Autodesk Inventor part; units mm, degrees
ref_plane "YZ Plane" through (0, 0, 0) normal (1, 0, 0) x (0, 1, 0)
ref_plane "XZ Plane" through (0, 0, 0) normal (0, 1, 0) x (-1, 0, 0)
ref_plane "XY Plane" through (0, 0, 0) normal (0, 0, 1) x (1, 0, 0)
sketch "Sketch1" plane through (0, 0, 0) normal (0, 0, 1) x (1, 0, 0)
  line L0 (-10.16, 7.62) -> (-15.748, 7.62)
  line L1 (-15.748, 7.62) -> (-15.748, 18.034)
  line L2 (-15.748, 18.034) -> (-23.368, 18.034)
  line L3 (-23.368, 18.034) -> (-23.368, 7.62)
  line L4 (-23.368, 7.62) -> (-105.283, 7.62)
  line L5 (-105.283, 7.62) -> (-105.283, 18.034)
  line L6 (-105.283, 18.034) -> (-112.903, 18.034)
  line L7 (-112.903, 18.034) -> (-112.903, 7.62)
  line L8 (-112.903, 7.62) -> (-123.571, 7.62)
  line L9 (-123.571, 7.62) -> (-123.571, 31.75)
  line L10 (-123.571, 31.75) -> (-133.731, 31.75)
  circle A0 centre (-109.093, 14.224) radius 1.778
  line L11 (-133.731, 31.75) -> (-133.731, 0)
  line L12 (-133.731, 0) -> (0, 0)
  circle A1 centre (-19.558, 14.224) radius 1.778
  line L13 (0, 0) -> (0, 20.32)
  line L14 (0, 20.32) -> (-10.16, 20.32)
  line L15 (-10.16, 20.32) -> (-10.16, 7.62)
  circle A2 centre (-128.143, 25.4) radius 2.413
  circle A3 centre (-63.5, 4.064) radius 2.413
  circle A4 centre (-5.6324, 15.2344) radius 2.413
  dimension "d22" = 20.32
  dimension "d39" = 4.826
  dimension "d40" = 4.826
  dimension "d41" = 4.826
extrude "Extrusion2" add sketch "Sketch1" along normal blind 13.081 contours L15 L14 L13 L12 L11 L10 L9 L8 L7 L6 L5 L4 L3 L2 L1 L0 | A2 | A3 | A4
sketch "Sketch2" plane through (0, 0, 0) normal (0, 0, 1) x (1, 0, 0)
  line L0 (-10.16, 7.62) -> (-15.748, 7.62)
  line L1 (-12.954, 7.62) -> (-118.4109, 7.62)
  line L2 (-118.4109, 7.62) -> (-118.4109, 21.3127)
  line L3 (-118.4109, 21.3127) -> (-12.954, 21.3127)
  line L4 (-12.954, 21.3127) -> (-12.954, 7.62)
  point P0 (0, 0)
extrude "Extrusion3" cut sketch "Sketch2" along normal blind 11.176
sketch "Sketch3" plane through (0, 0, 0) normal (1, 0, 0) x (0, 1, 0)
  line L0 (31.75, 13.081) -> (0, 13.081)
  line L1 (0.0413, 13.081) -> (0.0413, 28.575)
  line L2 (0.0413, 13.081) -> (15.5353, 13.081) construction
  line L3 (0.0413, 28.575) -> (10.2013, 28.575)
  line L4 (10.2013, 28.575) -> (10.2013, 13.081)
  circle A0 centre (5.1213, 24.8069) radius 1.778
  point P0 (0, 0)
  dimension "d28" = 15.494
  dimension "d29" = 90
  dimension "d30" = 10.16
  dimension "d31" = 3.556
extrude "Extrusion4" add sketch "Sketch3" against normal blind 2.032
ref_plane "Work Plane1" through (-133.731, 0, 0) normal (-1, 0, 0) x (0, 0, 1)
sketch "Sketch5" plane through (-133.731, 0, 0) normal (-1, 0, 0) x (0, 0, 1)
  line L0 (28.575, 10.2013) -> (13.081, 10.2013)
  line L1 (13.081, 0.0413) -> (28.575, 0.0413)
  line L2 (13.081, 10.2013) -> (28.575, 10.2013)
  line L3 (28.575, 10.2013) -> (28.575, 0.0413)
  line L4 (28.575, 0.0413) -> (13.081, 0.0413)
  line L5 (13.081, 0.0413) -> (13.081, 10.2013)
  circle A0 centre (24.7788, 5.1213) radius 1.778
  point P0 (0, 0)
  dimension "d36" = 3.556
extrude "Extrusion5" add sketch "Sketch5" against normal blind 2.032
ref_plane "Work Plane2" through (0, 0, 0) normal (0, 0, -1) x (-1, 0, 0)
sketch "Sketch6" plane through (0, 0, 0) normal (0, 0, -1) x (-1, 0, 0)
  circle A0 centre (5.588, 15.24) radius 2.413
  circle A1 centre (63.5, 4.0894) radius 2.286
  circle A2 centre (128.1176, 25.4) radius 2.413
  point P0 (0, 0)
  dimension "d43" = 4.826
  dimension "d44" = 4.572
  dimension "d45" = 4.826
extrude "Extrusion6" cut sketch "Sketch6" against normal blind 15.24
properties part number "PC_top_piece"
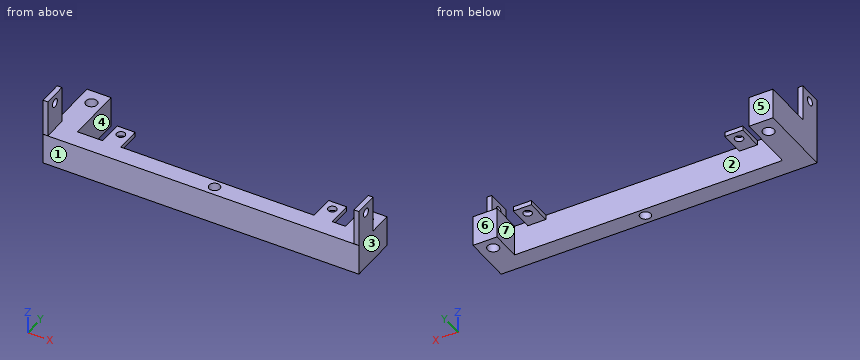
The model under review builds one solid part; all positions refer to its coordinate system, in mm. Face numbers are marked on the shaded views. A direction names the side the tool comes from. Coordinates: 2 decimals unless noted, no trailing zeros. Write each loop counter-clockwise with the first axis right and the second up, starting at its lowest first coordinate (ties: lowest second). Pieces come first, ordered by that corner, then holes. Notation, with made-up numbers: (-33, -7) - (-11, -7) arc R22 ccw to (-11, 7) - close; hole circle Ø7 at (49.5, 16). An arc over 180 degrees is marked (long way). Answer in a Markdown table with one row per item. Add a question column.
Q1. Consider section D-D on x = -41.5. Give the boundary of the cut face in (y, z).
Q2. Consider section B-B on z = 14.75. Give the boundary of the cut face in (x, y).
Q3. Consider section C-C on z = 7.5. Give the boundary of the cut face in (x, y), then the cut area to 3 significant figures.
Q4. To check wall thickness, follow line 1 along X through (y, z) = (1, 25.5); line 2 along X through (y, z) = (20.5, 2.25); line 3 along Z through (x, y) = (-12.5, 6). State the ranges of each line that lie inside material, in increasing order. Write a range as from..to.
Q5. Draft analysis for pull direction X (two halves, no side actions). For the marked faces 1, 2, 3 and 4, state which applies: +X half, -X half, draft (parallel to the pull), parting line (faces both ways), or undercut.
Q6. Clearance check with flat-ended pins moving along their axes: pin 1 (0.6 mm diameter, centred on x = -1, z = 21.5, fed in from +Y); pin 2 (2 mm diameter, centred on y = 24, z = 11, fed in from +X); pin 3 (1.5 mm diameter, centred on x = -109, z = 12, fed in from +Y). State where each tip first meets the part, or that it passes through.
Q7. For the marked faces 5, 6 and 7, list the 3-axis set-ups (+Z, -Z, +X, -X, +Y, -Y) from which the entire face can be reached by the end or side of a thin tool; tool diameter is ignored.
Q8. Consider section A-A on x = -63.5. Give the boundary of the cut face in (y, z), then the cut area to 3 significant figures.
Answers below:
| question | item | result |
|---|---|---|
| 1 | outline | (0, 0) - (7.62, 0) - (7.62, 13.08) - (0, 13.08) - close |
| 2 | outline | (-133.73, 0.04) - (-131.7, 0.04) - (-131.7, 10.2) - (-133.73, 10.2) - close; (-2.03, 0.04) - (0, 0.04) - (0, 10.2) - (-2.03, 10.2) - close |
| 3 | outline | (-133.73, 0) - (0, 0) - (0, 20.32) - (-10.16, 20.32) - (-10.16, 7.62) - (-123.57, 7.62) - (-123.57, 31.75) - (-133.73, 31.75) - close; hole circle Ø4.83 at (-128.12, 25.4); hole circle Ø4.57 at (-63.5, 4.09); hole circle Ø4.83 at (-5.59, 15.24) |
| 3 | area | 1,340 mm² |
| 4 | line 1 | -133.73..-131.7, -2.03..0 |
| 4 | line 2 | -133.73..-123.57 |
| 4 | line 3 | 0..13.08 |
| 5 | face 1 | draft |
| 5 | face 2 | undercut |
| 5 | face 3 | +X half |
| 5 | face 4 | undercut |
| 6 | pin 1 | y = 10.2 |
| 6 | pin 2 | x = -123.57 |
| 6 | pin 3 | y = 18.03 |
| 7 | face 5 | +Z, -Z, +X, -X, +Y |
| 7 | face 6 | +Z, -Z, +X, +Y |
| 7 | face 7 | +Z, -Z, +Y |
| 8 | outline | (0, 0) - (1.8, 0) - (1.8, 13.08) - (0, 13.08) - close; (6.38, 0) - (7.62, 0) - (7.62, 13.08) - (6.38, 13.08) - close |
| 8 | area | 39.9 mm² |
